```python
from build123d import *

# Parameters (mm, degrees)
SKETCH6_W           = 6.2
SKETCH6_H           = 6.2
BOSS_EXTRUDE4_DEPTH = 6.2
CUT_EXTRUDE3_DEPTH  = 1


with BuildPart() as part:
    # Sketch6 → Boss-Extrude4 (new body)
    with BuildSketch(Plane.XY):
        Polygon((157.908027241, 124.79254071), (153.794027241, 124.79254071), (153.794027241, 37.79254071), (132.344027241, 37.79254071), (132.344027241, 31.59254071), (126.144027241, 31.59254071), (126.144027241, 37.79254071), (119.944027241, 37.79254071), (119.944027241, 31.59254071), (113.744027241, 31.59254071), (113.744027241, 37.79254071), (77.544027241, 37.79254071), (77.544027241, -5.20745929), (182.594027241, -5.20745929), (182.594027241, 7.79254071), (188.794027241, 7.79254071), (188.794027241, 20.79254071), (182.594027241, 20.79254071), (182.594027241, 31.453899243), (176.394027241, 31.453899243), (176.394027241, 37.653899243), (182.594027241, 37.653899243), (182.594027241, 33.79254071), (188.794027241, 33.79254071), (188.794027241, 46.79254071), (182.594027241, 46.79254071), (182.594027241, 59.79254071), (188.794027241, 59.79254071), (188.794027241, 72.79254071), (182.594027241, 72.79254071), (182.594027241, 85.79254071), (188.794027241, 85.79254071), (188.794027241, 98.79254071), (182.594027241, 98.79254071), (182.594027241, 111.79254071), (188.794027241, 111.79254071), (188.794027241, 124.79254071), (178.478027241, 124.79254071), (178.478027241, 118.59254071), (174.364027241, 118.59254071), (174.364027241, 124.79254071), (170.250027241, 124.79254071), (170.250027241, 118.59254071), (166.136027241, 118.59254071), (166.136027241, 124.79254071), (162.022027241, 124.79254071), (162.022027241, 118.59254071), (157.908027241, 118.59254071), align=None)
        with Locations((167.094027241, 34.553899243)):
            Rectangle(SKETCH6_W, SKETCH6_H, mode=Mode.SUBTRACT)
    extrude(amount=BOSS_EXTRUDE4_DEPTH)

    # Sketch7 → Cut-Extrude3 (cut)
    with BuildSketch(Plane.XY.offset(6.2)):
        with BuildLine():
            Line((115.946331614, 11.576783669), (115.946331614, 11.251142644))
            Line((115.946331614, 11.251142644), (114.866373682, 11.251142644))
            Line((114.866373682, 11.251142644), (114.69528494, 10.416051498))
            add(Edge.make_bspline(
                [(114.69528494, 10.416051498), (114.728899911, 10.425331816), (114.794023603, 10.443310964), (114.890144334, 10.463273342), (114.981395832, 10.475306994), (115.040609919, 10.476950112), (115.069263305, 10.477745208)],
                knots=[0, 0, 0, 0, 0.000104595, 0.000202637, 0.000294305, 0.000380252, 0.000380252, 0.000380252, 0.000380252], degree=3))
            add(Edge.make_bspline(
                [(115.069263305, 10.477745208), (115.10471784, 10.476977823), (115.174430315, 10.475468954), (115.276428503, 10.460980204), (115.37379477, 10.43817471), (115.466325492, 10.40631538), (115.554191848, 10.365575836), (115.636585422, 10.314685176), (115.714742957, 10.255237083), (115.78726231, 10.186888393), (115.853052218, 10.111666641), (115.910897081, 10.030787715), (115.960030287, 9.945037622), (115.999546115, 9.853597069), (116.031100475, 9.75747698), (116.052102642, 9.655665995), (116.0660878, 9.549123772), (116.06765025, 9.476276054), (116.068446999, 9.439128421)],
                knots=[0, 0, 0, 0, 0.000106308, 0.000209029, 0.000308378, 0.000405929, 0.000502102, 0.000598312, 0.00069588, 0.000796219, 0.000896736, 0.000995218, 0.001094066, 0.001192613, 0.001293582, 0.001396995, 0.001504047, 0.001615439, 0.001615439, 0.001615439, 0.001615439], degree=3))
            add(Edge.make_bspline(
                [(116.068446999, 9.439128421), (116.067843681, 9.413254692), (116.066645197, 9.361856897), (116.060550479, 9.285526086), (116.048815936, 9.21081123), (116.033060929, 9.137702418), (116.012611736, 9.066338059), (115.987856666, 8.996513887), (115.957561698, 8.928664494), (115.924331807, 8.862147885), (115.886915359, 8.798467811), (115.845387713, 8.738914802), (115.801513304, 8.682595489), (115.754304332, 8.630113888), (115.703322001, 8.581814865), (115.649183746, 8.537411781), (115.592321565, 8.496153717), (115.531855738, 8.459715426), (115.469133628, 8.426184744), (115.40324946, 8.398676964), (115.335702967, 8.374083842), (115.265521973, 8.354480913), (115.192865443, 8.339120668), (115.117613611, 8.32868798), (115.040161146, 8.321089354), (114.987660242, 8.320613688), (114.961140308, 8.320373413)],
                knots=[0, 0, 0, 0, 7.7636e-05, 0.000154223, 0.000229512, 0.000304362, 0.000378447, 0.000452077, 0.000526407, 0.000601214, 0.00067506, 0.000747747, 0.00081887, 0.000889121, 0.000959302, 0.001029336, 0.001099058, 0.00116985, 0.001240974, 0.00131221, 0.00138383, 0.001456517, 0.001530612, 0.001606437, 0.001684346, 0.001763871, 0.001763871, 0.001763871, 0.001763871], degree=3))
            add(Edge.make_bspline(
                [(114.961140308, 8.320373413), (114.929504444, 8.321000102), (114.867264619, 8.322233038), (114.776078105, 8.335131235), (114.688344141, 8.353604216), (114.604768978, 8.38139569), (114.524603617, 8.41621845), (114.448927295, 8.460229548), (114.375806341, 8.51010345), (114.308213279, 8.568959198), (114.245478804, 8.633289853), (114.189320757, 8.703101427), (114.139306727, 8.777241707), (114.096237628, 8.856070747), (114.059500137, 8.939381414), (114.030639398, 9.02748585), (114.007345461, 9.119923711), (113.997490787, 9.183562967), (113.99248546, 9.215886233)],
                knots=[0, 0, 0, 0, 9.4843e-05, 0.000186593, 0.000275792, 0.000363484, 0.000450342, 0.000537514, 0.000625728, 0.000715478, 0.000805885, 0.000894984, 0.00098389, 0.001073836, 0.001164117, 0.001256635, 0.001351658, 0.001449737, 0.001449737, 0.001449737, 0.001449737], degree=3))
            Line((113.99248546, 9.215886233), (114.277421358, 9.215886233))
            add(Edge.make_bspline(
                [(114.277421358, 9.215886233), (114.284432264, 9.185609023), (114.297907613, 9.127414543), (114.327485686, 9.045652541), (114.36364973, 8.972791531), (114.406652246, 8.907867695), (114.457951202, 8.851253818), (114.516488613, 8.800801198), (114.582118333, 8.755285188), (114.655046477, 8.717345963), (114.731984056, 8.684989308), (114.812508596, 8.663443128), (114.894427539, 8.648293032), (114.949834347, 8.646776506), (114.977676767, 8.646014439)],
                knots=[0, 0, 0, 0, 9.3172e-05, 0.000179081, 0.000260145, 0.000336703, 0.000411917, 0.000488562, 0.000568128, 0.000650923, 0.00073478, 0.000817953, 0.000900557, 0.000983994, 0.000983994, 0.000983994, 0.000983994], degree=3))
            add(Edge.make_bspline(
                [(114.977676767, 8.646014439), (115.004853355, 8.646759001), (115.058364281, 8.648225052), (115.137114611, 8.659509013), (115.213144861, 8.676887667), (115.28570482, 8.702895321), (115.356064217, 8.734504458), (115.42244328, 8.77506742), (115.486762318, 8.821749008), (115.547022125, 8.875231094), (115.602212197, 8.934167888), (115.650976678, 8.997193809), (115.691595736, 9.064428377), (115.725825963, 9.134707595), (115.751818598, 9.208801714), (115.770361488, 9.286363495), (115.781249978, 9.367584512), (115.782747834, 9.4229831), (115.783511101, 9.451212756)],
                knots=[0, 0, 0, 0, 8.15e-05, 0.000160473, 0.000238226, 0.000315066, 0.000391338, 0.000469218, 0.000547964, 0.000629516, 0.000710512, 0.000789892, 0.000868102, 0.000945761, 0.001024012, 0.00110315, 0.001184644, 0.001269321, 0.001269321, 0.001269321, 0.001269321], degree=3))
            add(Edge.make_bspline(
                [(115.783511101, 9.451212756), (115.782913767, 9.476681473), (115.781744568, 9.526532864), (115.772191837, 9.59946643), (115.755575726, 9.668475547), (115.732512635, 9.733893459), (115.70323051, 9.795781868), (115.66744707, 9.854204644), (115.624490773, 9.908391764), (115.575421703, 9.95836858), (115.521666194, 10.004492145), (115.46229937, 10.043811424), (115.39856358, 10.076889406), (115.331226729, 10.105435376), (115.258687142, 10.125937481), (115.18238134, 10.141329777), (115.101485326, 10.150233713), (115.046176202, 10.15146914), (115.017745877, 10.152104182)],
                knots=[0, 0, 0, 0, 7.6388e-05, 0.000149519, 0.000220172, 0.000288967, 0.000357247, 0.000425206, 0.000494043, 0.000564207, 0.000635056, 0.000706145, 0.000777268, 0.000850264, 0.000925136, 0.001002969, 0.001083601, 0.001168886, 0.001168886, 0.001168886, 0.001168886], degree=3))
            add(Edge.make_bspline(
                [(115.017745877, 10.152104182), (114.993136063, 10.151577503), (114.942323041, 10.150490044), (114.864378762, 10.142483151), (114.782471271, 10.129566076), (114.69691455, 10.111798552), (114.60745166, 10.088547504), (114.514271397, 10.060685064), (114.417177841, 10.027372965), (114.351756762, 10.002215885), (114.318126486, 9.989283669)],
                knots=[0, 0, 0, 0, 7.3822e-05, 0.000152423, 0.000234822, 0.000322511, 0.00041445, 0.000512043, 0.000614219, 0.000722306, 0.000722306, 0.000722306, 0.000722306], degree=3))
            Line((114.318126486, 9.989283669), (114.643767512, 11.576783669))
            Line((114.643767512, 11.576783669), (115.946331614, 11.576783669))
        make_face()
        Polygon((118.127236061, 11.658193926), (118.185113666, 11.658193926), (118.185113666, 9.460117003), (118.551459819, 9.460117003), (118.551459819, 9.134475977), (118.185113666, 9.134475977), (118.185113666, 8.401783669), (117.900177768, 8.401783669), (117.900177768, 9.134475977), (116.394088025, 9.134475977), align=None)
        Polygon((117.900177768, 9.460117003), (117.900177768, 10.839003221), (116.953783537, 9.460117003), align=None, mode=Mode.SUBTRACT)
    extrude(amount=-CUT_EXTRUDE3_DEPTH, mode=Mode.SUBTRACT)


solid = part.part
```
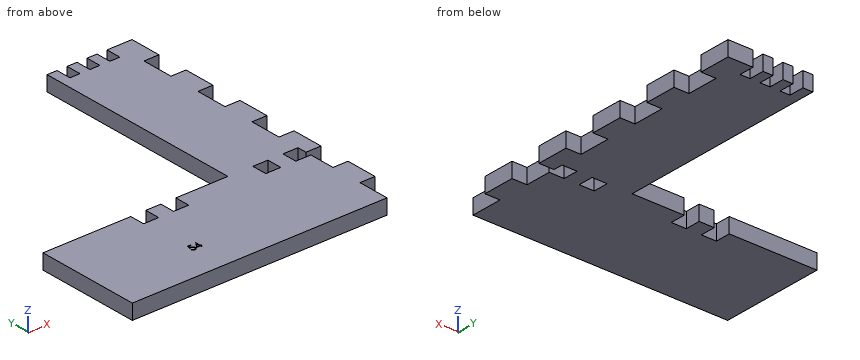
Verification items for the finished model (mm, model axes). Give positions to 0.01 mm unless a question says otherwise; leave off trailing zeros. Order: outer loops, then holes, each group sorted by start corner. A loop starts at its lowest first (then second) coordinate and runs counter-clockwise, first axis right, second up. Notation, with made-up numbers: (46, -10) -> (90, -10) arc R25 cw to (90, 9) -> close; hole circle Ø9 at (53.25, 22). An arc over 180 degrees is marked (long way). Use a Markdown table: item, result.
1) Material ranges on probe 1 along Y at (x, z) = (181, 1); probe 2 along X at (y, z) = (105, 0.75); probe 3 along Y at (x, z) = (126.5, 1), recorded low to high.
Results:
| item | result |
|---|---|
| probe 1 | -5.21 to 31.45, 37.65 to 124.79 |
| probe 2 | 153.79 to 182.59 |
| probe 3 | -5.21 to 31.59 |
2) Section check B-B, the plane y = 25.5. Record the boundary of the cut face in (x, z).
Results:
| item | result |
|---|---|
| outline | (77.54, 0) -> (182.59, 0) -> (182.59, 6.2) -> (77.54, 6.2) -> close |
3) Section check A-A, the plane x = 110.5. Record the boundary of the cut face in (y, z), then the cut area to 3 significant figures.
Results:
| item | result |
|---|---|
| outline | (-5.21, 0) -> (37.79, 0) -> (37.79, 6.2) -> (-5.21, 6.2) -> close |
| area | 267 mm² |
4) Depth check by flat-ended pin: pin 1 Ø3 at (y, z) = (105, 1) entering from +X; pin 2 Ø1.2 at (x, z) = (177, 2) entering from +Y; pin 3 Ø1.9 at (x, z) = (187, 3) entering from -Y. Enter the tip coordinate at first touch or a pass-through.
Results:
| item | result |
|---|---|
| pin 1 | x = 182.59 |
| pin 2 | y = 118.59 |
| pin 3 | y = 7.79 |
